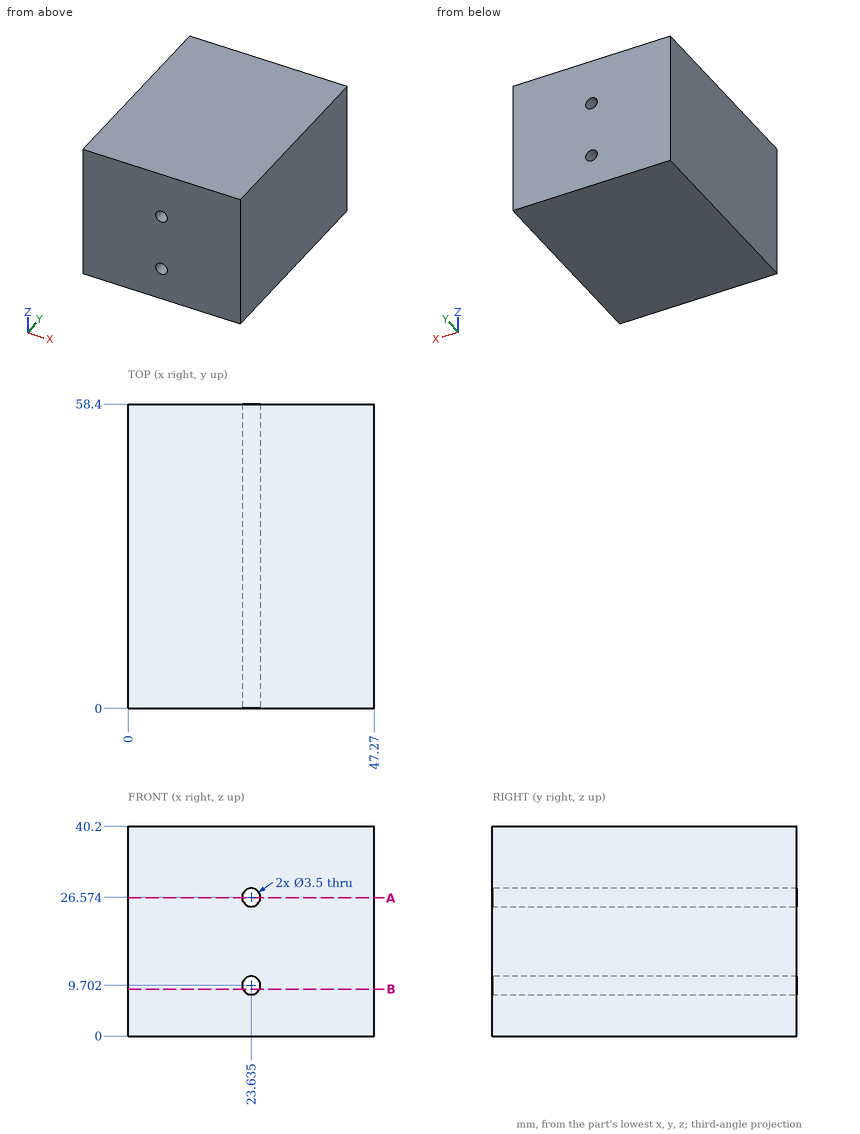
Geometry: see drawing. Coordinates: mm, zero at the bounding-box minimum. Round coordinates to 2 decimals unless told otherwise and drop trailing zeros. Write each loop counter-clockwise with the first axis right and the second up, starting at its lowest first coordinate (ties: lowest second). Pieces come first, ordered by that corner, then holes.
1) Cut plane B-B (z = 9). Return the cut outline in (x, y).
2) Cut plane A-A (z = 26.5). Return the cut outline in (x, y), then the cut area to 3 significant figures.
3) Ray query, L1, parallel to X at y = 36, z = 26; L2, parallel to X at y = 32, z = 9. Return the intervals inside material, ascending.
Geometry says:
1. outline: (0, 0) - (22.03, 0) - (22.03, 58.4) - (0, 58.4) - close; (25.24, 0) - (47.27, 0) - (47.27, 58.4) - (25.24, 58.4) - close
2. outline: (0, 0) - (21.89, 0) - (21.89, 58.4) - (0, 58.4) - close; (25.38, 0) - (47.27, 0) - (47.27, 58.4) - (25.38, 58.4) - close
2. area: 2,560 mm2
3. L1: x = 0 to 21.98, 25.29 to 47.27
3. L2: x = 0 to 22.03, 25.24 to 47.27
